CAD build for the part. Positions are in the model's coordinates, mm. A direction names the side the tool comes from. Give positions to 0.01 mm unless a question says otherwise; leave off trailing zeros. Write each loop counter-clockwise with the first axis right and the second up, starting at its lowest first coordinate (ties: lowest second). Pieces come first, ordered by that corner, then holes. Notation, with made-up numbers: (0, -34) - (38, -34) arc R28 cw to (38, -14) - close; hole circle Ø4 at (7, -27.5). An arc over 180 degrees is marked (long way). Put each result on its own line as item: value. Start each with the question number.
1. Wall check: line 1 (X direction, y = 10.75, z = -64); line 2 (Z direction, x = 26, y = 7.5); line 3 (X direction, y = 9.25, z = -7). Give the ranges that are in metal, low to high.
2. Cut at A-A on z = -31. List the corners of the cut face in (x, y), and give its area (3 significant figures).
3. Drop flat-ended pins along their axis: pin 1 (5 mm diameter, centred on x = 63.5, z = -52, fed in from -Y); pin 2 (1 mm diameter, centred on x = 34.5, y = 12, fed in from +Z). Give the stop position or say it passes through.
4. Cut at B-B on y = 10.5. List the corners of the cut face in (x, z) (3 decimals), and give its area (3 significant figures).
5. Cut at D-D on y = 1.5. Give the number of separate pieces and of enclosed holes in the cut face, and give its area (3 significant figures).
6. Cut at C-C on x = 57. List the corners of the cut face in (y, z).
7. Tool access for faces 1 (the flat face through (76.2, 7, -38)), 2 (the cylindrical face through (70.017, 6.261, -71.678)): list every direction of +Z, -Z, +X, -X, +Y, -Y with a clear straight run to the whole face (end or side of a thin tool).
8. Mould opens along Z. For faces 3 (the flat face through (3.81, 6, -39)), 4 (the flat face through (39, 7, -76.2)), 5 (the flat face through (38, 13.97, -39)) say: +Z half, -Z half, draft (parallel to the pull), parting line (faces both ways), or undercut.
Autodesk Inventor part; units mm, degrees
ref_plane "YZ Plane" through (0, 0, 0) normal (1, 0, 0) x (0, 1, 0)
ref_plane "XZ Plane" through (0, 0, 0) normal (0, 1, 0) x (-1, 0, 0)
ref_plane "XY Plane" through (0, 0, 0) normal (0, 0, 1) x (1, 0, 0)
sketch "Sketch1" plane through (0, 0, 0) normal (0, 1, 0) x (-1, 0, 0)
  line L0 (0, 0) -> (-76.2, 0)
  line L1 (-76.2, 0) -> (-76.2, -76.2)
  line L2 (-76.2, -76.2) -> (0, -76.2)
  line L3 (0, -76.2) -> (0, 0)
  line L4 (-8.89, -8.89) -> (-67.31, -8.89)
  line L5 (-67.31, -8.89) -> (-67.31, -67.31)
  line L6 (-67.31, -67.31) -> (-8.89, -67.31)
  line L7 (-8.89, -67.31) -> (-8.89, -8.89)
  line L8 (-8.89, -8.89) -> (-67.31, -67.31) construction
  line L9 (-67.31, -8.89) -> (-8.89, -67.31) construction
  point P0 (-38.1, -38.1)
  dimension "d0" = 76.2
  dimension "d1" = 76.2
  dimension "d2" = 58.42
  dimension "d3" = 58.42
extrude "Extrusion1" add sketch "Sketch1" along normal blind 12.7
sketch "Sketch2" plane through (0, 12.7, 0) normal (0, 1, 0) x (1, 0, 0)
  line L0 (0, 76.2) -> (0, 0)
  line L1 (76.2, 0) -> (76.2, 76.2)
  line L2 (0, 0) -> (76.2, 0)
  line L3 (76.2, 0) -> (76.2, 76.2)
  line L4 (76.2, 76.2) -> (0, 76.2)
  line L5 (0, 76.2) -> (0, 0)
extrude "Extrusion2" add sketch "Sketch2" along normal blind 1.27
sketch "Sketch3" plane through (0, 0, 0) normal (0, -1, 0) x (1, 0, 0)
  line L0 (67.31, -67.31) -> (67.31, -8.89) construction
  line L1 (76.2, 0) -> (76.2, -76.2) construction
  line L2 (67.31, -8.89) -> (76.2, 0) construction
  line L3 (67.31, -67.31) -> (76.2, -76.2) construction
  line L4 (8.89, -67.31) -> (0, -76.2) construction
  line L5 (8.89, -8.89) -> (8.89, -67.31) construction
  line L6 (8.89, -8.89) -> (0, 0) construction
  circle A0 centre (71.755, -4.445) radius 1.7399
  circle A1 centre (71.755, -71.755) radius 1.7399
  circle A2 centre (4.445, -4.445) radius 1.7399
  circle A3 centre (4.445, -71.755) radius 1.7399
  dimension "d8" = 3.4798
  dimension "d9" = 3.4798
  dimension "d10" = 3.4798
  dimension "d11" = 3.4798
extrude "Extrusion3" cut sketch "Sketch3" against normal blind 12.7
sketch "Sketch4" plane through (0, 0, 0) normal (0, -1, 0) x (1, 0, 0)
  line L0 (67.31, -67.31) -> (67.31, -8.89)
  line L1 (67.31, -8.89) -> (72.39, -8.89)
  line L2 (72.39, -8.89) -> (72.39, -67.31)
  line L3 (72.39, -67.31) -> (67.31, -67.31)
  line L4 (67.31, -67.31) -> (67.31, -8.89)
  circle A0 centre (38.1, -38.1) radius 2.0553 construction
  line L5 (8.89, -3.81) -> (67.31, -3.81)
  line L6 (8.89, -8.89) -> (8.89, -3.81)
  line L7 (67.31, -8.89) -> (8.89, -8.89)
  line L8 (67.31, -3.81) -> (67.31, -8.89)
  line L9 (3.81, -67.31) -> (3.81, -8.89)
  line L10 (8.89, -67.31) -> (3.81, -67.31)
  line L11 (8.89, -8.89) -> (8.89, -67.31)
  line L12 (3.81, -8.89) -> (8.89, -8.89)
  line L13 (67.31, -72.39) -> (8.89, -72.39)
  line L14 (67.31, -67.31) -> (67.31, -72.39)
  line L15 (8.89, -67.31) -> (67.31, -67.31)
  line L16 (8.89, -72.39) -> (8.89, -67.31)
  point P0 (0, 0)
  dimension "d14" = 5.08
  dimension "d17" = 360
extrude "Extrusion4" cut sketch "Sketch4" against normal blind 12.7 contours L0 L1 L2 L3 | L14 L13 L16 L15 | L7 L6 L5 L8 | L10 L9 L12 L11
sketch "Sketch5" plane through (0, 0, 0) normal (0, -1, 0) x (1, 0, 0)
  line L0 (0, 0) -> (76.2, 0)
  line L1 (47.85, 0) -> (28.35, 0)
  line L2 (28.35, 0) -> (28.35, -1.5)
  line L3 (28.35, -1.5) -> (38.1, -1.5)
  line L4 (47.85, -1.5) -> (47.85, 0)
  line L5 (8.89, -3.81) -> (67.31, -3.81) construction
  line L6 (38.1, -3.81) -> (38.1, 0) construction
  line L7 (48.1, -3.81) -> (28.1, -3.81)
  line L8 (28.1, -3.81) -> (28.1, -1.5)
  line L9 (48.1, -1.5) -> (48.1, -3.81)
  line L10 (28.1, -1.5) -> (38.1, -1.5)
  line L11 (47.85, -1.5) -> (48.1, -1.5)
  point P0 (28.35, 0)
  dimension "d21" = 19.5
  dimension "d22" = 1.5
  dimension "d23" = 20
extrude "Extrusion5" cut sketch "Sketch5" against normal blind 12.7
sketch "Sketch6" plane through (0, 0, 0) normal (0, -1, 0) x (1, 0, 0)
  line L0 (0, -76.2) -> (0, 0)
  line L1 (0, -33.85) -> (1, -33.85)
  line L2 (1, -33.85) -> (1, -42.35)
  line L3 (1, -42.35) -> (0, -42.35)
  line L4 (0, -42.35) -> (0, -33.85)
  line L5 (3.81, -67.31) -> (3.81, -8.89) construction
  line L6 (3.81, -38.1) -> (0, -38.1) construction
  line L7 (3.81, -29.35) -> (1, -29.35)
  line L8 (1, -29.35) -> (1, -46.85)
  line L9 (1, -46.85) -> (3.81, -46.85)
  line L10 (3.81, -46.85) -> (3.81, -29.35)
  dimension "d26" = 1
  dimension "d27" = 8.5
  dimension "d28" = 17.5
extrude "Extrusion6" cut sketch "Sketch6" against normal blind 4
sketch "Sketch7" plane through (0, 4, 0) normal (0, -1, 0) x (1, 0, 0)
  line L0 (1, -33.85) -> (1, -29.35)
  line L1 (0, -76.2) -> (0, -42.35)
  line L2 (1, -33.85) -> (0, -33.85)
  line L3 (0, -33.85) -> (0, -42.35)
  line L4 (0, -42.35) -> (1, -42.35)
  line L5 (1, -42.35) -> (1, -33.85)
  point P0 (0, 0)
extrude "Extrusion7" add sketch "Sketch7" along normal blind 1.5
properties part number "keypad cover good"
Report:
1. line 1: x = 0 to 3.81, 72.39 to 76.2
1. line 2: z = -76.2 to -72.39, -3.81 to 0
1. line 3: x = 0 to 8.89, 67.31 to 76.2
2. outline: (0, 0) - (1, 0) - (1, 4) - (3.81, 4) - (3.81, 12.7) - (72.39, 12.7) - (72.39, 0) - (76.2, 0) - (76.2, 13.97) - (0, 13.97) - close
2. area: 182 mm²
3. pin 1: stops at y = 12.7
3. pin 2: stops at z = -72.39
4. outline: (0, -76.2) - (76.2, -76.2) - (76.2, 0) - (47.85, 0) - (47.85, -1.5) - (48.1, -1.5) - (48.1, -3.81) - (67.31, -3.81) - (67.31, -8.89) - (72.39, -8.89) - (72.39, -67.31) - (67.31, -67.31) - (67.31, -72.39) - (8.89, -72.39) - (8.89, -67.31) - (3.81, -67.31) - (3.81, -8.89) - (8.89, -8.89) - (8.89, -3.81) - (28.1, -3.81) - (28.1, -1.5) - (28.35, -1.5) - (28.35, 0) - (0, 0) - close; hole circle Ø3.48 at (4.445, -71.755); hole circle Ø3.48 at (4.445, -4.445); hole circle Ø3.48 at (71.755, -71.755); hole circle Ø3.48 at (71.755, -4.445)
4. area: 1,090 mm²
5. separate pieces: 2
5. enclosed holes: 4
5. area: 1,040 mm²
6. outline: (0, -76.2) - (13.97, -76.2) - (13.97, 0) - (0, 0) - (0, -3.81) - (12.7, -3.81) - (12.7, -72.39) - (0, -72.39) - close
7. face 1: +Z, -Z, +X, +Y, -Y
7. face 2: -Y
8. face 3: undercut
8. face 4: -Z half
8. face 5: draft
